Design review of the part shown in the three views and the two pictorial views. Dimensions are in mm from the part's minimum x, y and z. Coordinates: 2 decimals unless noted, no trailing zeros. Loops run counter-clockwise (first coordinate to the right, second up) from the corner with the lowest first, then second, coordinate; pieces in that order, holes last. Notation, with made-up numbers: (72.25, 14.5) -> (81.25, 14.5) arc R17 cw to (81.25, 35.5) -> close; hole circle Ø8 at (20.25, -5.5). An arc over 180 degrees is marked (long way). Use a Markdown table: item, result. Add a question column.
Q1. Take a section at D-D on y = 0.9. Count the separate pieces of the cut face and the enclosed holes in it, plus the area to 3 significant figures.
Q2. For probe 1 along Z at (x, y) = (8.78, 0.45); probe 2 along Z at (x, y) = (42.78, 0.9); probe 3 along X at (y, z) = (0.9, 79.5), list the stretches that pass through material, from the lowest coordinate up.
Q3. Take a section at B-B on x = 8.78. Write out the cut boundary in (y, z), plus the area to 3 significant figures.
Q4. Take a section at A-A on x = 78.5. Write out the cut boundary in (y, z), plus the area to 3 significant figures.
Q5. Clearance check with flat-ended pins moving along their axes: pin 1 Ø4 at (x, z) = (84.78, 2.5) entering from -Y; pin 2 Ø0.8 at (x, y) = (25.5, 1) entering from -Z. State where each tip first meets the part, or that it passes through.
Q6. Take a section at C-C on z = 37. Write out the cut boundary in (x, y).
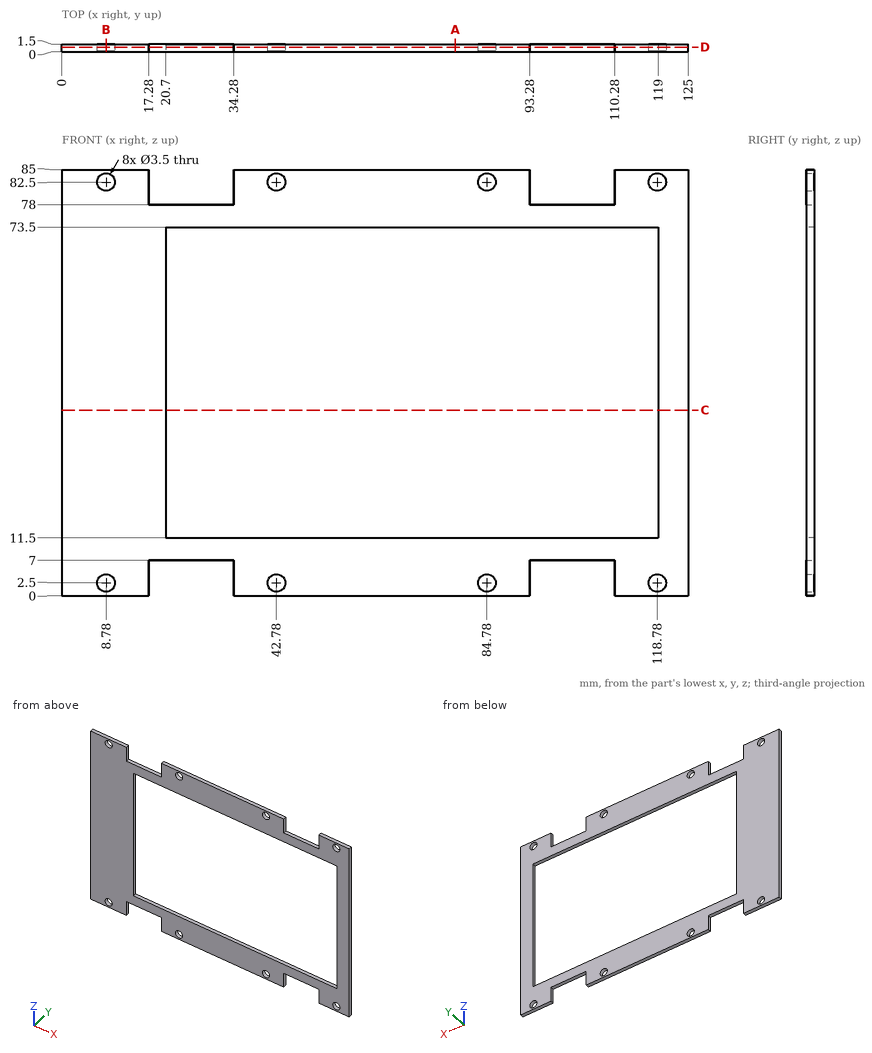
Answer list:
| question | item | result |
|---|---|---|
| 1 | separate pieces | 1 |
| 1 | enclosed holes | 9 |
| 1 | area | 3,980 mm² |
| 2 | probe 1 | 0 to 0.75, 4.25 to 80.75, 84.25 to 85 |
| 2 | probe 2 | 0 to 0.75, 4.25 to 11.5, 73.5 to 80.75, 84.25 to 85 |
| 2 | probe 3 | 0 to 17.28, 34.28 to 93.28, 110.28 to 125 |
| 3 | outline | (0, 0) -> (1.5, 0) -> (1.5, 0.75) -> (0, 0.75) -> close; (0, 4.25) -> (1.5, 4.25) -> (1.5, 80.75) -> (0, 80.75) -> close; (0, 84.25) -> (1.5, 84.25) -> (1.5, 85) -> (0, 85) -> close |
| 3 | area | 117 mm² |
| 4 | outline | (0, 0) -> (1.5, 0) -> (1.5, 11.5) -> (0, 11.5) -> close; (0, 73.5) -> (1.5, 73.5) -> (1.5, 85) -> (0, 85) -> close |
| 4 | area | 34.5 mm² |
| 5 | pin 1 | y = 0 |
| 5 | pin 2 | z = 7 |
| 6 | outline | (0, 0) -> (20.7, 0) -> (20.7, 1.5) -> (0, 1.5) -> close; (119, 0) -> (125, 0) -> (125, 1.5) -> (119, 1.5) -> close |
